The model under review builds one solid part; all positions refer to its coordinate system, in mm. A direction names the side the tool comes from. Coordinates: 2 decimals unless noted, no trailing zeros. Write each loop counter-clockwise with the first axis right and the second up, starting at its lowest first coordinate (ties: lowest second). Pieces come first, ordered by that corner, then holes. Notation, with made-up numbers: (49.25, 9) -> (98.25, 9) arc R35 ccw to (98.25, 42) -> close; hole circle Ø3 at (74, 24.5). An arc over 180 degrees is marked (long way). Put each result on its own line as item: value. Start each with the question number.
from build123d import *

# Parameters (mm, degrees)
SKETCH1_W                 = 6.35
SKETCH1_H                 = 38.1
BOSS_EXTRUDE1_DEPTH       = 175
M4X0_7_TAPPED_HOLE1_D     = 3.3
M4X0_7_TAPPED_HOLE1_DEPTH = 10.1
M4X0_7_TAPPED_HOLE1_TIP   = 0.991420021
M3X0_5_TAPPED_HOLE1_D     = 2.5
SKETCH9_W                 = 6.35
SKETCH9_H                 = 175
BOSS_EXTRUDE2_DEPTH       = 6.35
SKETCH8_R                 = 2.25
CUT_EXTRUDE1_DEPTH        = 181.668550113
M4X0_7_TAPPED_HOLE2_D     = 3.3
M4X0_7_TAPPED_HOLE2_DEPTH = 25.4
M4X0_7_TAPPED_HOLE2_TIP   = 0.991420021


with BuildPart() as part:
    # Sketch1 → Boss-Extrude1 (new body)
    with BuildSketch(Plane(origin=(0, 0, 0), x_dir=(1, 0, 0), z_dir=(0, 1, 0))):
        with Locations((3.175, 19.05)):
            Rectangle(SKETCH1_W, SKETCH1_H)
    extrude(amount=BOSS_EXTRUDE1_DEPTH)

    # M4x0.7 Tapped Hole1
    with Locations(Plane(origin=(0, 175, 0), x_dir=(1, 0, 0), z_dir=(0, 1, 0))):
        with Locations((3.175, 31.75), (3.175, 6.35)):
            Hole(M4X0_7_TAPPED_HOLE1_D / 2, depth=M4X0_7_TAPPED_HOLE1_DEPTH)
            with Locations((0, 0, -(M4X0_7_TAPPED_HOLE1_DEPTH + M4X0_7_TAPPED_HOLE1_TIP / 2))):  # 118° drill point
                Cone(0, M4X0_7_TAPPED_HOLE1_D / 2, M4X0_7_TAPPED_HOLE1_TIP, mode=Mode.SUBTRACT)

    # M3x0.5 Tapped Hole1 (through all)
    with Locations(Plane(origin=(6.35, 0, 0), x_dir=(0, 0, -1), z_dir=(1, 0, 0))):
        with Locations((19.05, 121.2), (19.05, 95.8), (19.05, 70.4), (19.05, 45), (19.05, 146.6)):
            Hole(M3X0_5_TAPPED_HOLE1_D / 2)

    # Sketch9 → Boss-Extrude2 (add)
    with BuildSketch(Plane(origin=(6.35, 0, 0), x_dir=(0, 0, -1), z_dir=(1, 0, 0))):
        with Locations((-3.175, 87.5)):
            Rectangle(SKETCH9_W, SKETCH9_H)
        with Locations((41.275, 87.5)):
            Rectangle(SKETCH9_W, SKETCH9_H)
    extrude(amount=-BOSS_EXTRUDE2_DEPTH)

    # Sketch8 → Cut-Extrude1 (cut, through all)
    with BuildSketch(Plane(origin=(6.35, 0, 0), x_dir=(0, 0, -1), z_dir=(1, 0, 0))):
        with Locations((36.524, 33.675)):
            Circle(SKETCH8_R)
        with Locations((1.524, 33.675)):
            Circle(SKETCH8_R)
    extrude(amount=-CUT_EXTRUDE1_DEPTH, mode=Mode.SUBTRACT)

    # M4x0.7 Tapped Hole2
    with Locations(Plane(origin=(0, 0, 0), x_dir=(-1, 0, 0), z_dir=(0, -1, 0))):
        with Locations((-3.175, 6.35), (-3.175, 31.75)):
            Hole(M4X0_7_TAPPED_HOLE2_D / 2, depth=M4X0_7_TAPPED_HOLE2_DEPTH)
            with Locations((0, 0, -(M4X0_7_TAPPED_HOLE2_DEPTH + M4X0_7_TAPPED_HOLE2_TIP / 2))):  # 118° drill point
                Cone(0, M4X0_7_TAPPED_HOLE2_D / 2, M4X0_7_TAPPED_HOLE2_TIP, mode=Mode.SUBTRACT)


solid = part.part
1. Tool access review of faces 1 (the cylindrical face through (3.53, 169.88, -4.74)), 2 (the cylindrical face through (2.96, 12.878, -33.386)), 3 (the cylindrical face through (3.219, 32.306, -34.738)): name each direction out of +Z, -Z, +X, -X, +Y, -Y from which nothing blocks a thin tool from reaching the whole face with its end or side.
2. Consider section A-A on y = 12. State the section outline as (x, z) points (3 decimals), then the cut area to 3 significant figures.
3. Wall thickness on line 1 (Z direction, x = 5.25, y = 95.5); line 2 (X direction, y = 11, z = -6.35) (3 decimals); line 3 (Z direction, x = 4, y = 35): over which ranges is each line inside the solid? List them lowest first. Write a range as from..to.
4. Insertion check: P1, Ø3, axis at x = 3.175, z = -6.35, coming from the +Y side; P2, Ø2.5, axis at x = 3.175, z = -31.75, coming from the +Y side; P3, Ø1.5, axis at y = 146.6, z = -19.05, coming from the +X side. Each pin has a flat end and moves straight along its axis. Give the tip position at first contact, or say it passes through.
5. The part is to be moulded in two halves that separate along Z. For faces 4 (the flat face through (3, 86, -44.45)), 5 (the flat face through (3, 175, -19)), 6 (the flat face through (3, 86, 6.35)), 7 (the cylindrical face through (3.39, 169.879, -33.386)), say which applies: released by +Z, released by -Z, zero draft, split by the parting line, or undercut.
Output values:
1. face 1: +Y
1. face 2: -Y
1. face 3: +X, -X
2. outline: (0, -44.45) -> (6.35, -44.45) -> (6.35, 6.35) -> (0, 6.35) -> close; hole circle Ø3.3 at (3.175, -31.75); hole circle Ø3.3 at (3.175, -6.35)
2. area: 305 mm^2
3. line 1: z = -44.45..-20.26, -17.84..6.35
3. line 2: x = 0..1.525, 4.825..6.35
3. line 3: z = -44.45..-38.34, -34.71..-3.34, 0.29..6.35
4. P1: stops at y = 164.81
4. P2: stops at y = 164.66
4. P3: passes through
5. face 4: released by -Z
5. face 5: zero draft
5. face 6: released by +Z
5. face 7: undercut
